Design review of the part built by this model. Coordinates are the model's own, in mm. A direction names the side the tool comes from. Coordinates: 2 decimals unless noted, no trailing zeros. Order: outer loops, then holes, each group sorted by start corner. A loop starts at its lowest first (then second) coordinate and runs counter-clockwise, first axis right, second up. Notation, with made-up numbers: (60, 69.25) - (106, 69.25) arc R18 ccw to (106, 88.25) - close; hole circle Ø1 at (21, 89). An arc over 180 degrees is marked (long way). Write item = value, one per line. Start each with the question number.
```python
from build123d import *

# Parameters (mm, degrees)
SKETCH1_W               = 27.0002
SKETCH1_H               = 25.9842
BOSS_EXTRUDE1_DEPTH     = 5.08
SKETCH2_R               = 1.9939
SKETCH2_R_2             = 1.6383
BOSS_EXTRUDE2_DEPTH     = 11.4808
SKETCH3_R               = 1.641593419
SKETCH3_R_2             = 1.6383
CUT_EXTRUDE1_DEPTH      = 1
CUT_EXTRUDE1_DEPTH_BACK = 17.5608


with BuildPart() as part:
    # Sketch1 → Boss-Extrude1 (new body)
    with BuildSketch(Plane(origin=(0, 0, 0), x_dir=(1, 0, 0), z_dir=(0, 1, 0))):
        with Locations((2.217200719, -2.362930935)):
            Rectangle(SKETCH1_W, SKETCH1_H)
    extrude(amount=BOSS_EXTRUDE1_DEPTH)

    # Sketch2 → Boss-Extrude2 (add)
    with BuildSketch(Plane.XZ):
        with Locations((-9.082699611, 13.17672836)):
            Circle(SKETCH2_R)
        with Locations((-9.082699611, 13.17672836)):
            Circle(SKETCH2_R_2, mode=Mode.SUBTRACT)
        with Locations((13.612727851, 13.17672836)):
            Circle(SKETCH2_R)
        with Locations((13.612727851, 13.17672836)):
            Circle(SKETCH2_R_2, mode=Mode.SUBTRACT)
        with Locations((-9.082699611, -8.403053089)):
            Circle(SKETCH2_R)
        with Locations((-9.082699611, -8.403053089)):
            Circle(SKETCH2_R_2, mode=Mode.SUBTRACT)
        with Locations((13.612727851, -8.403053089)):
            Circle(SKETCH2_R)
        with Locations((13.612727851, -8.403053089)):
            Circle(SKETCH2_R_2, mode=Mode.SUBTRACT)
    extrude(amount=BOSS_EXTRUDE2_DEPTH)

    # Sketch3 → Cut-Extrude1 (cut, two sides)
    with BuildSketch(Plane(origin=(0, 5.08, 0), x_dir=(1, 0, 0), z_dir=(0, 1, 0))) as cut_extrude1_sk:
        with Locations((13.612727851, 8.403053089)):
            Circle(SKETCH3_R)
        with Locations((-9.082699611, 8.403053089)):
            Circle(SKETCH3_R_2)
        with Locations((13.612727851, -13.17672836)):
            Circle(SKETCH3_R_2)
        with Locations((-9.082699611, -13.17672836)):
            Circle(SKETCH3_R_2)
    extrude(amount=CUT_EXTRUDE1_DEPTH, mode=Mode.SUBTRACT)
    extrude(cut_extrude1_sk.sketch, amount=-CUT_EXTRUDE1_DEPTH_BACK, mode=Mode.SUBTRACT)


solid = part.part
```
Item 1: Add section D-D on z = 4.25. Give the boundary of the cut face in (x, y).
Item 2: Mouldability with a two-part tool opening along Z and no side actions: class faces 3 (the flat face through (-9, -11.481, 15)), 4 (the cylindrical face through (12.405, -3.084, 12.069)), 5 (the flat face through (2, 3, 15.355)) as +Z half, -Z half, draft (parallel to the pull), parting line (faces both ways), or undercut.
Item 3: For line 1 (X direction, y = -0.75, z = -8.5); line 2 (Z direction, x = -9.75, y = -2.5); line 3 (X direction, y = -5.75, z = 13.75), list the stretches that pass through material, from the lowest coordinate up.
Item 4: Add section B-B on y = 2.75. Give the boundary of the cut face in (x, z).
Item 5: Add section A-A on y = -9.5. Give the boundary of the cut face in (x, z).
Item 6: Add section C-C on x = 1. Give the boundary of the cut face in (y, z), plus the area to 3 significant figures.
Item 7: For P1, Ø1.5, axis at y = -5.5, z = -7.5, coming from the +X side; P2, Ø1, axis at x = 8.5, z = 1, coming from the -Y side, all flat-tipped, find the tip position at first contact; note any pin that passes through.
Item 8: For faces 1 (the cylindrical face through (11.62, -5.66, 13.26)), 2 (the flat face through (2, 5.08, 2)), list the 3-axis set-ups (+Z, -Z, +X, -X, +Y, -Y) from which the entire face can be reached by the end or side of a thin tool; tool diameter is ignored.
Worked out:
q1.outline = (-11.28, 0) - (15.72, 0) - (15.72, 5.08) - (-11.28, 5.08) - close
q2.face_3 = draft
q2.face_4 = undercut
q2.face_5 = +Z half
q3.line_1 = -11.07 to -10.72, -7.45 to -7.09, 11.62 to 11.97, 15.25 to 15.6
q3.line_2 = -10.28 to -9.9, -6.91 to -6.52, 11.3 to 11.68, 14.67 to 15.06
q3.line_3 = -10.99 to -10.62, -7.55 to -7.17, 11.7 to 12.08, 15.15 to 15.52
q4.outline = (-11.28, -10.63) - (15.72, -10.63) - (15.72, 15.36) - (-11.28, 15.36) - close; hole circle Ø3.28 at (-9.08, -8.4); hole circle Ø3.28 at (-9.08, 13.18); hole circle Ø3.28 at (13.61, -8.4); hole circle Ø3.28 at (13.61, 13.18)
q5.outline = circle Ø3.99 at (-9.08, -8.4); circle Ø3.99 at (-9.08, 13.18); circle Ø3.99 at (13.61, -8.4); circle Ø3.99 at (13.61, 13.18); hole circle Ø3.28 at (-9.08, -8.4); hole circle Ø3.28 at (-9.08, 13.18); hole circle Ø3.28 at (13.61, -8.4); hole circle Ø3.28 at (13.61, 13.18)
q6.outline = (0, -10.63) - (5.08, -10.63) - (5.08, 15.36) - (0, 15.36) - close
q6.area = 132 mm2
q7.P1 = 15.6
q7.P2 = 0
q8.face_1 = -Y
q8.face_2 = +Z, -Z, +X, -X, +Y
